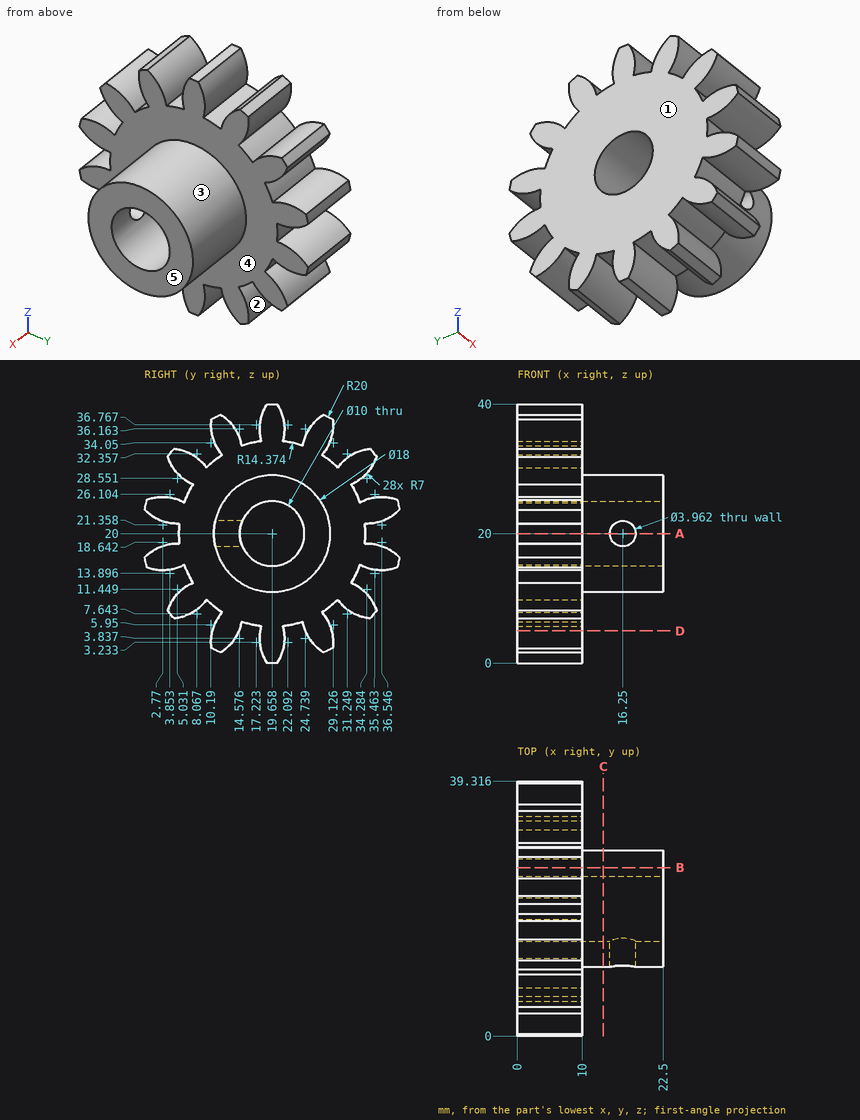
Source: three-view drawing plus pictorial views. Frame: mm from the lowest corner of the part. A direction names the side the tool comes from. Coordinates: 2 decimals unless noted, no trailing zeros. Write each loop counter-clockwise with the first axis right and the second up, starting at its lowest first coordinate (ties: lowest second). Pieces come first, ordered by that corner, then holes. Notation, with made-up numbers: (19, 44) -> (44, 44) arc R21 ccw to (44, 73) -> close; hole circle Ø1 at (75, -17.5). An arc over 180 degrees is marked (long way). Answer as a JSON object with one key per item and string values.
1. Section C-C on x = 13.25. Return the cut outline in (y, z).
Result set:
{"outline": "circle Ø18 at (19.66, 20); hole circle Ø10 at (19.66, 20)"}
2. Access query for the marked faces 4 and 5. Directions: +Z, -Z, +X, -X, +Y, -Y. A direction counts if a zero-diameter tool reaches every point of the face in a straight line with its end or side. Return the directions, or none.
Result set:
{"face 4": "+X", "face 5": "+Z, -Z, +X, +Y, -Y"}
3. Section A-A on z = 20. Return the cut outline in (x, y).
Result set:
{"outline": "(0, 5.28) -> (10, 5.28) -> (10, 10.66) -> (14.27, 10.66) -> (14.27, 14.66) -> (0, 14.66) -> close; (0, 24.66) -> (22.5, 24.66) -> (22.5, 28.66) -> (10, 28.66) -> (10, 34.03) -> (0, 34.03) -> close; (18.23, 10.66) -> (22.5, 10.66) -> (22.5, 14.66) -> (18.23, 14.66) -> close"}
4. First-contact query: P1, Ø3, axis at x = 10, z = 9, coming from the +Y side; P2, Ø8, axis at x = 16, z = 9.5, coming from the +Y side; P3, Ø5, axis at x = 16.25, z = 20, coming from the +Y side. Flat tips, straight axial feed; report the tip coordinate or a pass-through.
Result set:
{"P1": "stops at y = 35.77", "P2": "stops at y = 25.88", "P3": "stops at y = 28.66"}
5. Section D-D on z = 5. Count the separate pieces of the cut face and the enclosed holes in it, then the cut area to 3 significant figures.
Result set:
{"separate pieces": "3", "enclosed holes": "0", "area": "118 mm2"}
6. Section B-B on y = 26. Return the cut outline in (x, z) (1 decimal).
Result set:
{"outline": "(0, 3) -> (10, 3) -> (10, 13.6) -> (22.5, 13.6) -> (22.5, 26.4) -> (10, 26.4) -> (10, 37) -> (0, 37) -> close"}
7. Mould query, pull axis Y, two halves, no side actions, for the marked faces 1, 2 and 3. Classes: released by +Y, released by -Y, zero draft, split by the parting line, or undercut.
Result set:
{"face 1": "zero draft", "face 2": "undercut", "face 3": "split by the parting line"}
8. Material intervals for line 1 (X direction, y = 12, z = 20); line 2 (Y direction, x = 8.5, z = 20); line 3 (Z direction, x = 8, y = 20), sorted ascending. Write a range as from..to.
Result set:
{"line 1": "x = 0..14.27, 18.23..22.5", "line 2": "y = 5.28..14.66, 24.66..34.03", "line 3": "z = 0..15.01, 24.99..40"}
